Design review of the part built by this model. Coordinates are the model's own, in mm. A direction names the side the tool comes from. Give positions to 0.01 mm unless a question says otherwise; leave off trailing zeros. Write each loop counter-clockwise with the first axis right and the second up, starting at its lowest first coordinate (ties: lowest second). Pieces come first, ordered by that corner, then holes. Notation, with made-up numbers: (18.5, 3) -> (73.5, 3) arc R25 ccw to (73.5, 28) -> close; hole circle Ø4 at (64, 58.5). An arc over 180 degrees is marked (long way). Write each question's results on one line, items separated by ' | '. Start each with the question number.
(1) Take a section at A-A (z = 23.75). State the section outline as (x, y) points.
(2) For faces 1 (the face through (-9, 16.261, 13)), 2 (the face through (-19, -2, 15.875)), 3 (the face through (-20.512, -26.805, 14.143)), 4 (the face through (-19, -1, 9.525)), list the 3-axis set-ups (+Z, -Z, +X, -X, +Y, -Y) from which the entire face can be reached by the end or side of a thin tool; tool diameter is ignored.
(3) Mouldability with a two-part tool opening along Y and no side actions: class faces 5 (the face through (-20.232, 28.7, 24.465)), 6 (the face through (-20, 35, 25.4)), 7 (the face through (-20.01, -19.49, 12.66)) as released by +Y, released by -Y, zero draft, split by the parting line, or undercut.
(4) Take a section at C-C (y = -10). State the section outline as (x, z) points (3 decimals).
(5) To check wall thickness, follow probe 1 along Y at (x, z) = (-20.5, 14); probe 2 along Z at (x, y) = (-13.5, 10.5) (3 decimals); probe 3 along X at (y, z) = (4, 12.75). State the ranges of each line that lie inside material, in increasing order.
(6) Clearance check with flat-ended pins moving along their axes: pin 1 (7 mm diameter, centred on y = -1, z = 12, fed in from +X); pin 2 (1.9 mm diameter, centred on x = -8.5, z = 14, fed in from +Y); pin 3 (1 mm diameter, centred on y = 31, z = 9.5, fed in from -X); pin 4 (5.5 mm diameter, centred on x = -20.31, y = 33.08, fed in from -Z). State where each tip first meets the part, or that it passes through.
(7) Take a section at B-B (x = -7.75). State the section outline as (y, z) points (3 decimals).
(8) Take a section at D-D (z = 12.7). State the section outline as (x, y) points (1 decimal).
from build123d import *

# Parameters (mm, degrees)
SKETCH1_W               = 22.225
SKETCH1_H               = 67.6402
BOSS_EXTRUDE1_DEPTH     = 25.4
SKETCH2_R               = 1.7907
CUT_EXTRUDE2_DEPTH      = 25.4
SKETCH4_W               = 9.525
SKETCH4_H               = 10.16
SKETCH4_H_2             = 35.894850391
SKETCH4_H_3             = 35.916644849
CUT_EXTRUDE3_DEPTH      = 51.712797865
SKETCH5_R               = 2.38125
CUT_EXTRUDE4_DEPTH      = 6.35
CUT_EXTRUDE5_REACH      = 79.582
CUT_EXTRUDE5_END_RADIUS = 2.38125
SKETCH6_R               = 1.455475959


with BuildPart() as part:
    # Sketch1 → Boss-Extrude1 (new body)
    with BuildSketch(Plane.XY):
        with Locations((-17.147623967, 4.03062314)):
            Rectangle(SKETCH1_W, SKETCH1_H)
    extrude(amount=BOSS_EXTRUDE1_DEPTH)

    # Sketch2 → Cut-Extrude2 (cut)
    with BuildSketch(Plane.XY.offset(25.4)):
        with BuildLine():
            ThreePointArc((-20.309923967, 37.85072314), (-16.933347665, 36.452099442), (-15.534723967, 33.07552314))
            Line((-15.534723967, 33.07552314), (-15.534723967, 31.988846816))
            ThreePointArc((-15.534723967, 31.988846816), (-15.164047916, 28.377221194), (-14.067475414, 24.916185349))
            Line((-14.067475414, 24.916185349), (-13.85237252, 24.420060932))
            ThreePointArc((-13.85237252, 24.420060932), (-12.755800018, 20.959025087), (-12.385123967, 17.347399465))
            Line((-12.385123967, 17.347399465), (-12.385123967, 16.26072314))
            Line((-12.385123967, 16.26072314), (-6.035123967, 16.26072314))
            Line((-6.035123967, 16.26072314), (-6.035123967, 37.85072314))
            Line((-6.035123967, 37.85072314), (-20.309923967, 37.85072314))
        make_face()
        with BuildLine():
            Line((-25.085123967, 32.016111722), (-25.085123967, 33.07552314))
            ThreePointArc((-25.085123967, 33.07552314), (-23.686500268, 36.452099442), (-20.309923967, 37.85072314))
            Line((-20.309923967, 37.85072314), (-28.260123967, 37.85072314))
            Line((-28.260123967, 37.85072314), (-28.260123967, 17.320134559))
            ThreePointArc((-28.260123967, 17.320134559), (-27.884120973, 20.957343409), (-26.772015056, 24.440716329))
            Line((-26.772015056, 24.440716329), (-26.573232878, 24.895529952))
            ThreePointArc((-26.573232878, 24.895529952), (-25.461126961, 28.378902872), (-25.085123967, 32.016111722))
        make_face()
        with BuildLine():
            Line((-6.035123967, -29.78947686), (-6.035123967, 6.10072314))
            Line((-6.035123967, 6.10072314), (-12.385123967, 6.10072314))
            Line((-12.385123967, 6.10072314), (-12.385123967, -21.85197686))
            ThreePointArc((-12.385123967, -21.85197686), (-14.709963891, -27.464636935), (-20.322623967, -29.78947686))
            Line((-20.322623967, -29.78947686), (-6.035123967, -29.78947686))
        make_face()
        with BuildLine():
            ThreePointArc((-20.322623967, -29.78947686), (-25.935284043, -27.464636935), (-28.260123967, -21.85197686))
            Line((-28.260123967, -21.85197686), (-28.260123967, -29.78947686))
            Line((-28.260123967, -29.78947686), (-20.322623967, -29.78947686))
        make_face()
        with Locations((-20.309923967, 33.07552314)):
            Circle(SKETCH2_R)
    extrude(amount=-CUT_EXTRUDE2_DEPTH, mode=Mode.SUBTRACT)

    # Sketch4 → Cut-Extrude3 (cut, through all)
    with BuildSketch(Plane(origin=(-6.035123967, 0, 0), x_dir=(0, 0, -1), z_dir=(1, 0, 0))):
        with BuildLine():
            Line((-9.525, 16.698464592), (-9.525, 16.26072314))
            Line((-9.525, 16.26072314), (0, 16.26072314))
            Line((0, 16.26072314), (0, 32.637781689))
            ThreePointArc((0, 32.637781689), (-0.909409772, 28.750457477), (-3.448884978, 25.669973531))
            Line((-3.448884978, 25.669973531), (-6.076115022, 23.66627275))
            ThreePointArc((-6.076115022, 23.66627275), (-8.615590228, 20.585788804), (-9.525, 16.698464592))
        make_face()
        with Locations((-4.7625, 11.18072314)):
            Rectangle(SKETCH4_W, SKETCH4_H)
        with Locations((-4.7625, -11.846702056)):
            Rectangle(SKETCH4_W, SKETCH4_H_2)
        with Locations((-20.6375, -11.857599285)):
            Rectangle(SKETCH4_W, SKETCH4_H_3)
        with Locations((-20.6375, 11.18072314)):
            Rectangle(SKETCH4_W, SKETCH4_H)
        with BuildLine():
            Line((-25.4, 16.26072314), (-15.875, 16.26072314))
            Line((-15.875, 16.26072314), (-15.875, 16.698464592))
            ThreePointArc((-15.875, 16.698464592), (-16.784409772, 20.585788804), (-19.323884978, 23.66627275))
            Line((-19.323884978, 23.66627275), (-21.951115022, 25.669973531))
            ThreePointArc((-21.951115022, 25.669973531), (-24.490590228, 28.750457477), (-25.4, 32.637781689))
            Line((-25.4, 32.637781689), (-25.4, 16.26072314))
        make_face()
    extrude(amount=-CUT_EXTRUDE3_DEPTH, mode=Mode.SUBTRACT)

    # Sketch5 → Cut-Extrude4 (cut)
    with BuildSketch(Plane(origin=(0, 0, 9.525), x_dir=(-1, 0, 0), z_dir=(0, 0, -1))):
        with Locations((20.322623967, -21.85197686)):
            Circle(SKETCH5_R)
    extrude(amount=-CUT_EXTRUDE4_DEPTH, mode=Mode.SUBTRACT)

    # Cut-Extrude5: up to this cylinder (the profile starts outside it)
    cut_extrude5_end = Plane(origin=(-20.322623967, -21.85197686, 12.7), z_dir=(0, 0, -1)) * Cylinder(CUT_EXTRUDE5_END_RADIUS, 164.9265, mode=Mode.PRIVATE)
    # Sketch6 → Cut-Extrude5 (cut, up to the surface)
    with BuildSketch(Plane.XZ.offset(29.78947686), mode=Mode.PRIVATE) as cut_extrude5_sk1:
        with Locations((-20.322623967, 12.7)):
            Circle(SKETCH6_R)
    cut_extrude5_tool1 = extrude(cut_extrude5_sk1.sketch, amount=-CUT_EXTRUDE5_REACH, mode=Mode.PRIVATE) - cut_extrude5_end
    add(cut_extrude5_tool1.solids().sort_by_distance((-20.322624, -29.789477, 12.7))[0], mode=Mode.SUBTRACT)


solid = part.part
Report:
1) outline: (-25.66, 27.52) -> (-14.96, 27.52) arc R17.78 cw to (-15.53, 31.99) -> (-15.53, 33.08) arc R4.78 ccw to (-25.09, 33.08) -> (-25.09, 32.02) arc R17.78 cw to start; hole circle Ø3.58 at (-20.31, 33.08)
2) face 1: +Z, -Z, +X, +Y | face 2: +Z, +X, -X, -Y | face 3: -Y | face 4: -Z, +X, -X, -Y
3) face 5: released by -Y | face 6: zero draft | face 7: undercut
4) outline: (-28.26, 9.525) -> (-12.385, 9.525) -> (-12.385, 15.875) -> (-28.26, 15.875) -> close
5) probe 1: -19.48 to 31.29, 34.86 to 37.85 | probe 2: 9.525 to 15.875 | probe 3: -28.26 to -12.39
6) pin 1: x = -12.39 | pin 2: y = 16.26 | pin 3: x = -25.15 | pin 4: z = 0
7) outline: (6.101, 9.525) -> (16.261, 9.525) -> (16.261, 15.875) -> (6.101, 15.875) -> close
8) outline: (-28.3, -21.9) arc R7.9 ccw to (-21.8, -29.7) -> (-21.8, -23.7) arc R2.4 cw (long way) to (-18.9, -23.7) -> (-18.9, -29.7) arc R7.9 ccw to (-12.4, -21.9) -> (-12.4, 6.1) -> (-6, 6.1) -> (-6, 16.3) -> (-12.4, 16.3) -> (-12.4, 17.3) arc R17.8 ccw to (-13.9, 24.4) -> (-14.1, 24.9) arc R17.8 cw to (-15.5, 32) -> (-15.5, 33.1) arc R4.8 ccw to (-25.1, 33.1) -> (-25.1, 32) arc R17.8 cw to (-26.6, 24.9) -> (-26.8, 24.4) arc R17.8 ccw to (-28.3, 17.3) -> close; hole circle Ø3.6 at (-20.3, 33.1)
